from build123d import *

# Parameters (mm, degrees)
SKETCH1_W           = 360
SKETCH1_H           = 90
SKETCH1_H_2         = 378
SKETCH1_W_2         = 220
SKETCH1_H_3         = 248
BOSS_EXTRUDE1_DEPTH = 8


with BuildPart() as part:
    # Sketch1 → Boss-Extrude1 (new body)
    # profile 1 of 2: a face of its own
    with BuildSketch(Plane.XY):
        with Locations((0, -239)):
            Rectangle(SKETCH1_W, SKETCH1_H)
    # profile 2 of 2: a face of its own
    with BuildSketch(Plane.XY):
        with Locations((0, -5)):
            Rectangle(SKETCH1_W, SKETCH1_H_2)
        Rectangle(SKETCH1_W_2, SKETCH1_H_3, mode=Mode.SUBTRACT)
    extrude(amount=BOSS_EXTRUDE1_DEPTH)


solid = part.part
Input: part model. Units: mm. Frame: model coordinates. Round coordinates to 2 decimals unless told otherwise and drop trailing zeros. Order: outer loops, then holes, each group sorted by start corner. A loop starts at its lowest first (then second) coordinate and runs counter-clockwise, first axis right, second up.
1. Cut plane A-A, the plane y = -110. Output: boundary loops of the cut face in (x, z).
The answers:
outline: (-180, 0) - (-110, 0) - (-110, 8) - (-180, 8) - close; (110, 0) - (180, 0) - (180, 8) - (110, 8) - close
2. Cut plane B-B, the plane x = 66.5. Output: boundary loops of the cut face in (y, z).
The answers:
outline: (-284, 0) - (-124, 0) - (-124, 8) - (-284, 8) - close; (124, 0) - (184, 0) - (184, 8) - (124, 8) - close
3. Material intervals for line 1 (X direction, y = -59.5, z = 1.5); line 2 (Y direction, x = 103.5, z = 5.5), sorted ascending.
The answers:
line 1: x = -180 to -110, 110 to 180
line 2: y = -284 to -124, 124 to 184
4. Cut plane C-C, the plane z = 1.5. Output: boundary loops of the cut face in (x, y), then the cut area to 3 significant figures.
The answers:
outline: (-180, -284) - (180, -284) - (180, 184) - (-180, 184) - close; hole (-110, -124) - (110, -124) - (110, 124) - (-110, 124) - close
area: 114,000 mm2
